Work out the finished part from the listing and answer in its coordinate system (mm). Coordinates: 2 decimals unless noted, no trailing zeros. Use one line per item in the form item = value.
from build123d import *

# Parameters (mm, degrees)
SKETCH1_R           = 2.6035
BOSS_EXTRUDE1_DEPTH = 119.38


with BuildPart() as part:
    # Sketch1 → Boss-Extrude1 (new, symmetric)
    with BuildSketch(Plane.XY):
        with BuildLine():
            Line((-7.179650497, -8.645192506), (-3.952270251, -5.423690499))
            ThreePointArc((-3.952270251, -5.423690499), (-2.922936451, -4.736929036), (-1.709253557, -4.4958))
            Line((-1.709253557, -4.4958), (1.709253557, -4.4958))
            ThreePointArc((1.709253557, -4.4958), (2.922936451, -4.736929036), (3.952270251, -5.423690499))
            Line((3.952270251, -5.423690499), (7.179650497, -8.645192506))
            ThreePointArc((7.179650497, -8.645192506), (7.41473083, -9.822813117), (6.416408329, -10.4902))
            Line((6.416408329, -10.4902), (4.287512407, -10.4902))
            ThreePointArc((4.287512407, -10.4902), (3.54574862, -10.79744862), (3.2385, -11.539212407))
            Line((3.2385, -11.539212407), (3.2385, -11.650987593))
            ThreePointArc((3.2385, -11.650987593), (3.54574862, -12.39275138), (4.287512407, -12.7))
            Line((4.287512407, -12.7), (5.317126718, -12.7))
            ThreePointArc((5.317126718, -12.7), (5.825126718, -12.192), (6.333126718, -12.7))
            Line((6.333126718, -12.7), (9.550443118, -12.7))
            ThreePointArc((9.550443118, -12.7), (10.058366869, -12.192000006), (10.566443095, -12.699847501))
            ThreePointArc((10.566443095, -12.699847501), (12.082537762, -12.08250727), (12.699846982, -10.566399977))
            ThreePointArc((12.699846982, -10.566399977), (12.192000006, -10.058323491), (12.7, -9.5504))
            Line((12.7, -9.5504), (12.7, -6.3330836))
            ThreePointArc((12.7, -6.3330836), (12.192, -5.8250836), (12.7, -5.3170836))
            Line((12.7, -5.3170836), (12.7, -4.287469289))
            ThreePointArc((12.7, -4.287469289), (12.39275138, -3.545705502), (11.650987593, -3.238456882))
            Line((11.650987593, -3.238456882), (11.539212407, -3.238456882))
            ThreePointArc((11.539212407, -3.238456882), (10.79744862, -3.545705502), (10.4902, -4.287469289))
            Line((10.4902, -4.287469289), (10.4902, -6.402089023))
            ThreePointArc((10.4902, -6.402089023), (9.856505071, -7.351067942), (8.737131347, -7.129408934))
            Line((8.737131347, -7.129408934), (5.441005833, -3.840816462))
            ThreePointArc((5.441005833, -3.840816462), (4.750877967, -2.809883091), (4.5085, -1.593185507))
            Line((4.5085, -1.593185507), (4.5085, 1.593185507))
            ThreePointArc((4.5085, 1.593185507), (4.750877967, 2.809883091), (5.441005833, 3.840816462))
            Line((5.441005833, 3.840816462), (8.737131347, 7.129408934))
            ThreePointArc((8.737131347, 7.129408934), (9.856505071, 7.351067942), (10.4902, 6.402089023))
            Line((10.4902, 6.402089023), (10.4902, 4.287469289))
            ThreePointArc((10.4902, 4.287469289), (10.79744862, 3.545705502), (11.539212407, 3.238456882))
            Line((11.539212407, 3.238456882), (11.650987593, 3.238456882))
            ThreePointArc((11.650987593, 3.238456882), (12.39275138, 3.545705502), (12.7, 4.287469289))
            Line((12.7, 4.287469289), (12.7, 5.3170836))
            ThreePointArc((12.7, 5.3170836), (12.192, 5.8250836), (12.7, 6.3330836))
            Line((12.7, 6.3330836), (12.7, 9.5504))
            ThreePointArc((12.7, 9.5504), (12.192000006, 10.058323491), (12.699846982, 10.566399977))
            ThreePointArc((12.699846982, 10.566399977), (12.082537762, 12.08250727), (10.566443095, 12.699847501))
            ThreePointArc((10.566443095, 12.699847501), (10.058366869, 12.192000006), (9.550443118, 12.7))
            Line((9.550443118, 12.7), (6.333126718, 12.7))
            ThreePointArc((6.333126718, 12.7), (5.825126718, 12.192), (5.317126718, 12.7))
            Line((5.317126718, 12.7), (4.287512407, 12.7))
            ThreePointArc((4.287512407, 12.7), (3.54574862, 12.39275138), (3.2385, 11.650987593))
            Line((3.2385, 11.650987593), (3.2385, 11.539212407))
            ThreePointArc((3.2385, 11.539212407), (3.54574862, 10.79744862), (4.287512407, 10.4902))
            Line((4.287512407, 10.4902), (6.476788598, 10.4902))
            ThreePointArc((6.476788598, 10.4902), (7.432222385, 9.85140422), (7.207036008, 8.724370562))
            Line((7.207036008, 8.724370562), (3.898272566, 5.423169045))
            ThreePointArc((3.898272566, 5.423169045), (2.869120213, 4.736787962), (1.655778399, 4.4958))
            Line((1.655778399, 4.4958), (-1.655778399, 4.4958))
            ThreePointArc((-1.655778399, 4.4958), (-2.869120213, 4.736787962), (-3.898272566, 5.423169045))
            Line((-3.898272566, 5.423169045), (-7.207036008, 8.724370562))
            ThreePointArc((-7.207036008, 8.724370562), (-7.432222385, 9.85140422), (-6.476788598, 10.4902))
            Line((-6.476788598, 10.4902), (-4.287512407, 10.4902))
            ThreePointArc((-4.287512407, 10.4902), (-3.54574862, 10.79744862), (-3.2385, 11.539212407))
            Line((-3.2385, 11.539212407), (-3.2385, 11.650987593))
            ThreePointArc((-3.2385, 11.650987593), (-3.54574862, 12.39275138), (-4.287512407, 12.7))
            Line((-4.287512407, 12.7), (-5.317126718, 12.7))
            ThreePointArc((-5.317126718, 12.7), (-5.825126718, 12.192), (-6.333126718, 12.7))
            Line((-6.333126718, 12.7), (-9.550443118, 12.7))
            ThreePointArc((-9.550443118, 12.7), (-10.058366869, 12.192000006), (-10.566443095, 12.699847501))
            ThreePointArc((-10.566443095, 12.699847501), (-12.082537762, 12.08250727), (-12.699846982, 10.566399977))
            ThreePointArc((-12.699846982, 10.566399977), (-12.192000006, 10.058323491), (-12.7, 9.5504))
            Line((-12.7, 9.5504), (-12.7, 6.3330836))
            ThreePointArc((-12.7, 6.3330836), (-12.192, 5.8250836), (-12.7, 5.3170836))
            Line((-12.7, 5.3170836), (-12.7, 4.287469289))
            ThreePointArc((-12.7, 4.287469289), (-12.39275138, 3.545705502), (-11.650987593, 3.238456882))
            Line((-11.650987593, 3.238456882), (-11.539212407, 3.238456882))
            ThreePointArc((-11.539212407, 3.238456882), (-10.79744862, 3.545705502), (-10.4902, 4.287469289))
            Line((-10.4902, 4.287469289), (-10.4902, 6.402089023))
            ThreePointArc((-10.4902, 6.402089023), (-9.856505071, 7.351067942), (-8.737131347, 7.129408934))
            Line((-8.737131347, 7.129408934), (-5.441005833, 3.840816462))
            ThreePointArc((-5.441005833, 3.840816462), (-4.750877967, 2.809883091), (-4.5085, 1.593185507))
            Line((-4.5085, 1.593185507), (-4.5085, -1.593185507))
            ThreePointArc((-4.5085, -1.593185507), (-4.750877967, -2.809883091), (-5.441005833, -3.840816462))
            Line((-5.441005833, -3.840816462), (-8.737131347, -7.129408934))
            ThreePointArc((-8.737131347, -7.129408934), (-9.856505071, -7.351067942), (-10.4902, -6.402089023))
            Line((-10.4902, -6.402089023), (-10.4902, -4.287469289))
            ThreePointArc((-10.4902, -4.287469289), (-10.79744862, -3.545705502), (-11.539212407, -3.238456882))
            Line((-11.539212407, -3.238456882), (-11.650987593, -3.238456882))
            ThreePointArc((-11.650987593, -3.238456882), (-12.39275138, -3.545705502), (-12.7, -4.287469289))
            Line((-12.7, -4.287469289), (-12.7, -5.3170836))
            ThreePointArc((-12.7, -5.3170836), (-12.192, -5.8250836), (-12.7, -6.3330836))
            Line((-12.7, -6.3330836), (-12.7, -9.5504))
            ThreePointArc((-12.7, -9.5504), (-12.192000006, -10.058323491), (-12.699846982, -10.566399977))
            ThreePointArc((-12.699846982, -10.566399977), (-12.082537762, -12.08250727), (-10.566443095, -12.699847501))
            ThreePointArc((-10.566443095, -12.699847501), (-10.058366869, -12.192000006), (-9.550443118, -12.7))
            Line((-9.550443118, -12.7), (-6.333126718, -12.7))
            ThreePointArc((-6.333126718, -12.7), (-5.825126718, -12.192), (-5.317126718, -12.7))
            Line((-5.317126718, -12.7), (-4.287512407, -12.7))
            ThreePointArc((-4.287512407, -12.7), (-3.54574862, -12.39275138), (-3.2385, -11.650987593))
            Line((-3.2385, -11.650987593), (-3.2385, -11.539212407))
            ThreePointArc((-3.2385, -11.539212407), (-3.54574862, -10.79744862), (-4.287512407, -10.4902))
            Line((-4.287512407, -10.4902), (-6.416408329, -10.4902))
            ThreePointArc((-6.416408329, -10.4902), (-7.41473083, -9.822813117), (-7.179650497, -8.645192506))
        make_face()
        with Locations(Location((0, 0, 0), (0, 0, 180))):
            Circle(SKETCH1_R, mode=Mode.SUBTRACT)
    extrude(amount=BOSS_EXTRUDE1_DEPTH, both=True)


solid = part.part
(1) The mould has two halves that part along Y. Classify faces 1 (the flat face through (3, 0, 119.38)), 2 (the cylindrical face through (-2.483, -0.782, -1.671)): released by +Y, released by -Y, zero draft, split by the parting line, or undercut.
Data:
face_1 = zero draft
face_2 = undercut
(2) Each of these flat-tipped pins is pushed along its axis until it touches: P1, Ø1, axis at y = 0, z = -12.5, coming from the +X side; P2, Ø1.5, axis at y = -4, z = -87, coming from the -X side; P3, Ø1.7, axis at x = 0, z = -4.5, coming from the +Y side; P4, Ø3.5, axis at y = -0.5, z = -56.5, coming from the +X side. Where does it stop, or does it pass through?
Data:
P1 = 4.51
P2 = -12.7
P3 = 4.5
P4 = 4.58
(3) Straight lines are drawn through the part: line 1 along Y through (x, z) = (0.5, 29); line 2 along X through (y, z) = (2, -43.5); line 3 along X through (y, z) = (-6.5, -100.5). For each, find the intervals that lie inside material, in ascending order.
Data:
line_1 = -4.5 to -2.56, 2.56 to 4.5
line_2 = -4.53 to -1.67, 1.67 to 4.53
line_3 = -12.7 to -10.49, -8.11 to -5.03, 5.03 to 8.11, 10.49 to 12.7
